```python
from build123d import *

# Parameters (mm, degrees)
F1_DEPTH = 17
F2_R     = 1


with BuildPart() as f1:
    # F0 (on Front) → F1 (new body)
    with BuildSketch(Plane.XZ):
        with BuildLine():
            ThreePointArc((7.5, 9), (17.742641, 13.242641), (13.5, 3))
            Line((13.5, 3), (2, 3))
            ThreePointArc((2, 3), (0.585786, 2.414214), (0, 1))
            Line((0, 1), (0, 0))
            Line((0, 0), (28, 0))
            Line((28, 0), (28, 1))
            ThreePointArc((28, 1), (27.414214, 2.414214), (26, 3))
            Line((26, 3), (22.665151, 3))
            ThreePointArc((22.665151, 3), (20.991831, 3.904555), (20.832121, 5.8))
            ThreePointArc((20.832121, 5.8), (15.691096, 16.694095), (5.582053, 10.142857))
            ThreePointArc((5.582053, 10.142857), (5.815868, 9.345346), (6.571797, 9))
            Line((6.571797, 9), (7.5, 9))
        make_face()
    extrude(amount=F1_DEPTH)

    # F2
    f2_edges = [f1.edges().sort_by_distance(p)[0] for p in [
        (7.75, 0, 3),
        (17.742641, -17, 13.242641),
    ]]
    fillet(f2_edges, radius=F2_R)


solid = f1.part
```
Geometry check sheet. Reference: the model listing, model coordinates, mm. A direction names the side the tool comes from. Coordinates: 2 decimals unless noted, no trailing zeros. Order: outer loops, then holes, each group sorted by start corner. A loop starts at its lowest first (then second) coordinate and runs counter-clockwise, first axis right, second up.
Item 1: Mould release check, pull along Z, two halves, no side actions. Record for faces 5 (the flat face through (15, -17, 2)), 6 (the cylindrical face through (7.67, -16.699, 2.715)), 7 (the cylindrical face through (27.43, -8.38, 2.4)): released by +Z, released by -Z, zero draft, split by the parting line, or undercut.
Item 2: Scan lines: line 1 along Z through (x, y) = (13.5, -8); line 2 along Z through (x, y) = (22.5, -1.75); line 3 along Z through (x, y) = (12.75, -0.5). Record each from-to range of solid material in increasing order.
Item 3: Depth check by flat-ended pin: pin 1 (1.7 mm diameter, centred on x = 25, y = -5, fed in from +Z); pin 2 (6 mm diameter, centred on y = -14, z = 15, fed in from +X); pin 3 (1.5 mm diameter, centred on y = -4.5, z = 12, fed in from -X). Enter the tip coordinate at first touch or a pass-through.
Item 4: Tool access check on faces 1 (the flat face through (0, -8.4, 0.5)), 2 (the flat face through (24, -8, 3)), 3 (the cylindrical face through (7.67, -0.301, 2.715)), 4 (the flat face through (8, -8, 3)). Record the directions out of +Z, -Z, +X, -X, +Y, -Y that give a thin tool (end or side, any length) a straight path to the whole face; none if there is none.
Item 5: Section check A-A (y = -13.25). Enter the section's corners in (x, z), plus the area to 3 significant figures.
Check sheet entries:
1. face 5: zero draft
1. face 6: undercut
1. face 7: released by +Z
2. line 1: z = 0 to 3, 15 to 17
2. line 2: z = 0 to 3.01
2. line 3: z = 0 to 2.87, 15.09 to 16.96
3. pin 1: stops at z = 3
3. pin 2: stops at x = 20.92
3. pin 3: stops at x = 5.82
4. face 1: +Z, -Z, -X, +Y, -Y
4. face 2: +Z, +X, +Y, -Y
4. face 3: -X, +Y
4. face 4: -X, +Y, -Y
5. outline: (0, 0) - (28, 0) - (28, 1) arc R2 ccw to (26, 3) - (22.67, 3) arc R2 cw to (20.83, 5.8) arc R8 ccw (long way) to (5.58, 10.14) arc R1 ccw to (6.57, 9) - (7.5, 9) arc R6 cw (long way) to (13.5, 3) - (2, 3) arc R2 ccw to (0, 1) - close
5. area: 144 mm2
